Check sheet for the drawn part. Datum: minimum x, y, z corner. Units: mm. A direction names the side the tool comes from. Give positions to 0.01 mm unless a question says otherwise; leave off trailing zeros. Loops run counter-clockwise (first coordinate to the right, second up) from the corner with the lowest first, then second, coordinate; pieces in that order, holes last. Notation, with made-up numbers: (77, -2.5) - (102, -2.5) arc R17 ccw to (102, 30.5) - close; hole circle Ø11 at (-20.5, 53.5). An arc over 180 degrees is marked (long way). Use one line per item in the form item = value.
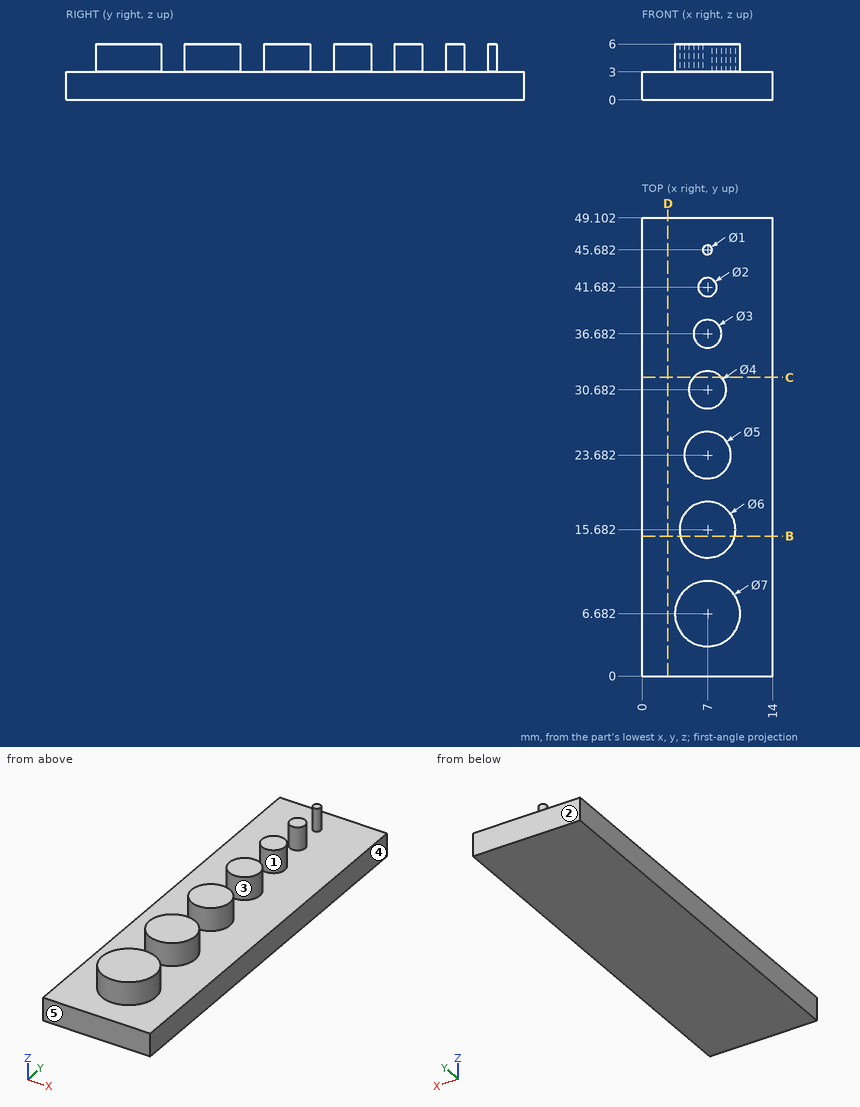
Item 1: Thickness scan on L1, parallel to X at y = 6.5, z = 4.2 (1 decimal); L2, parallel to Z at x = 12, y = 36; L3, parallel to X at y = 23, z = 4.65 (1 decimal). Record the ranges inside material, lowest first.
Answer block:
L1 = 3.5 to 10.5
L2 = 0 to 3
L3 = 4.6 to 9.4
Item 2: Section check D-D on x = 2.75. Record the boundary of the cut face in (y, z), then the cut area to 3 significant figures.
Answer block:
outline = (0, 0) - (49.1, 0) - (49.1, 3) - (0, 3) - close
area = 147 mm2
Item 3: Mould release check, pull along Y, two halves, no side actions. Record for the marked faces 3, 4 and 5: released by +Y, released by -Y, zero draft, split by the parting line, or undercut.
Answer block:
face_3 = undercut
face_4 = zero draft
face_5 = released by -Y
Item 4: Section check B-B on y = 15. Record the boundary of the cut face in (x, z).
Answer block:
outline = (0, 0) - (14, 0) - (14, 3) - (9.92, 3) - (9.92, 6) - (4.08, 6) - (4.08, 3) - (0, 3) - close
Item 5: Access from +Z, -Z, +X, -X, +Y, -Y to the whole of each face (thin tool, end or side, straight path). Record for the marked faces 1 and 2.
Answer block:
face_1 = +Z
face_2 = +Z, -Z, +X, -X, +Y
Item 6: Gauge pin test, flat ends, axial feed: P1, Ø3, axis at x = 7.5, z = 5, coming from the -Y side; P2, Ø1, axis at y = 13, z = 4, coming from the -X side. Record the tip position at first contact, or that the pin passes through.
Answer block:
P1 = 3.18
P2 = 4.94
Item 7: Section check C-C on y = 32. Record the boundary of the cut face in (x, z).
Answer block:
outline = (0, 0) - (14, 0) - (14, 3) - (8.5, 3) - (8.5, 6) - (5.5, 6) - (5.5, 3) - (0, 3) - close
